Input: part model. Units: mm. Frame: model coordinates. Round coordinates to 2 decimals unless told otherwise and drop trailing zeros. One line per item, written item: value. Start each with the question number.
Autodesk Inventor part; units mm, degrees
ref_plane "YZ Plane" through (0, 0, 0) normal (1, 0, 0) x (0, 1, 0)
ref_plane "XZ Plane" through (0, 0, 0) normal (0, 1, 0) x (-1, 0, 0)
ref_plane "XY Plane" through (0, 0, 0) normal (0, 0, 1) x (1, 0, 0)
sketch "Sketch1" plane through (0, 0, 0) normal (0, 0, 1) x (1, 0, 0)
  line L0 (-277, -354.5) -> (277, -354.5)
  line L1 (277, -354.5) -> (277, 354.5)
  line L2 (277, 354.5) -> (-277, 354.5)
  line L3 (-277, 354.5) -> (-277, -354.5)
  line L4 (-277, -354.5) -> (277, 354.5) construction
  line L5 (277, -354.5) -> (-277, 354.5) construction
  line L6 (0, 0) -> (0, 354.5) construction
  line L7 (250, 311.5) -> (-250, 311.5) construction
  line L8 (-250, 311.5) -> (-250, 339.5) construction
  line L9 (-250, 339.5) -> (250, 339.5) construction
  line L10 (250, 339.5) -> (250, 311.5) construction
  line L11 (250, 311.5) -> (-250, 339.5) construction
  line L12 (-250, 311.5) -> (250, 339.5) construction
  point P0 (0, 325.5)
  point P1 (0, 311.5)
  point P2 (0, 339.5)
  dimension "d0" = 554
  dimension "d1" = 709
  dimension "d4" = 500
  dimension "d5" = 28
  dimension "d6" = 15
extrude "Extrusion1" add sketch "Sketch1" along normal blind 18
hole "Hole1" at (-250, 311.5, 0) at (-250, 339.5, 0) at (0, 311.5, 0) at (0, 339.5, 0) at (250, 339.5, 0) at (250, 311.5, 0) direction (0, 0, 1) diameter 3 depth 8 tip angle 118
pattern_linear "Rectangular Pattern1" count 2 spacing 550 along (0, -1, 0) of "Hole1"
properties part number "wozek_podstawa"
Q1. Contact query for flat-ended pins moving along their axis: pin 1 Ø4 at (x, y) = (250, -210.5) entering from -Z; pin 2 Ø2.5 at (x, y) = (250, 339.5) entering from -Z; pin 3 Ø1.8 at (x, y) = (-250, 339.5) entering from -Z. Output: stop coordinate, or through.
Q2. Material intervals for probe 1 along Y at (x, z) = (250, 4.75); probe 2 along X at (y, z) = (311.5, 6), sorted ascending. Write a range as from..to.
Q3. Pull-direction query (X, two-part tool) for faces 1 (the flat face through (-4, 5, 0)), 2 (the flat face through (277, -5, 9)), 3 (the flat face through (-277, 5, 9)); classes: pulls with the +X half, pulls with the -X half, needs draft (parallel to the pull), parting line crosses it, or undercut.
A:
1. pin 1: stops at z = 0
1. pin 2: stops at z = 8.15
1. pin 3: stops at z = 8.36
2. probe 1: y = -354.5..-240, -237..-212, -209..310, 313..338, 341..354.5
2. probe 2: x = -277..-251.5, -248.5..-1.5, 1.5..248.5, 251.5..277
3. face 1: needs draft
3. face 2: pulls with the +X half
3. face 3: pulls with the -X half
